Could you check a few things on this model? Use its own coordinates, in mm. A direction names the side the tool comes from. Round coordinates to 2 decimals unless told otherwise and drop trailing zeros. Loops run counter-clockwise (first coordinate to the right, second up) from the corner with the lowest first, then second, coordinate; pieces in that order, holes last.
from build123d import *

# Parameters (mm, degrees)
SKETCH_W        = 160
SKETCH_H        = 160
PAD_DEPTH       = 10
SKETCH001_R     = 80
SKETCH001_R_2   = 64
POCKET_DEPTH    = 5
SKETCH002_R     = 3.1
POCKET001_DEPTH = 10
SKETCH003_R     = 10
PAD001_DEPTH    = 10
SKETCH004_R     = 3.1
POCKET002_DEPTH = 14


with BuildPart() as part:
    # Sketch → Pad (new body)
    with BuildSketch(Plane.XY):
        with Locations((80, 80)):
            Rectangle(SKETCH_W, SKETCH_H)
    extrude(amount=PAD_DEPTH)

    # Sketch001 (on Face6 of Pad) → Pocket (cut)
    with BuildSketch(Plane.XY.offset(10)):
        with Locations((48, 48)):
            Circle(SKETCH001_R)
        with Locations((48, 48)):
            Circle(SKETCH001_R_2, mode=Mode.SUBTRACT)
    extrude(amount=-POCKET_DEPTH, mode=Mode.SUBTRACT)

    # Sketch002 (on Face5 of Pocket) → Pocket001 (cut)
    with BuildSketch(Plane.XY.offset(10)):
        with Locations((20, 140)):
            Circle(SKETCH002_R)
        with Locations((80, 140)):
            Circle(SKETCH002_R)
        with Locations((140, 140)):
            Circle(SKETCH002_R)
        with Locations((140, 80)):
            Circle(SKETCH002_R)
        with Locations((140, 20)):
            Circle(SKETCH002_R)
    extrude(amount=-POCKET001_DEPTH, mode=Mode.SUBTRACT)

    # Sketch003 (on Face9 of Pocket001) → Pad001 (join)
    with BuildSketch(Plane.XY.offset(10)):
        with Locations((48, 48)):
            Circle(SKETCH003_R)
    extrude(amount=PAD001_DEPTH)

    # Sketch004 (on Face21 of Pad001) → Pocket002 (cut)
    with BuildSketch(Plane.XY.offset(20)):
        with Locations((48, 48)):
            Circle(SKETCH004_R)
    extrude(amount=-POCKET002_DEPTH, mode=Mode.SUBTRACT)


solid = part.part
Item 1: We'd pull the mould along X, two halves only. Please class faces 1 (the cylindrical face through (142.957, 20.931, 5.07)), 2 (the flat face through (114, 117, 10)), 3 (the cylindrical face through (2.71, 2.78, 7.54)): released by +X, released by -X, zero draft, split by the parting line, or undercut.
Results list:
face 1: undercut
face 2: zero draft
face 3: released by -X
Item 2: Will these pins go through, and if not, where does the flat tip stop? pin 1 (7 mm diameter, centred on x = 49, y = 48, fed in from +Z); pin 2 (8 mm diameter, centred on x = 20, y = 140, fed in from +Z); pin 3 (1 mm diameter, centred on y = 56.5, z = 14.5, fed in from +X); pin 4 (5 mm diameter, centred on x = 140, y = 80, fed in from +Z).
Results list:
pin 1: stops at z = 20
pin 2: stops at z = 10
pin 3: stops at x = 54
pin 4: passes through
Item 3: If we section it at D-D, the plane x = 80: Please give me the cut outline in (y, z).
Results list:
outline: (0, 0) - (136.9, 0) - (136.9, 10) - (121.32, 10) - (121.32, 5) - (103.43, 5) - (103.43, 10) - (0, 10) - close; (143.1, 0) - (160, 0) - (160, 10) - (143.1, 10) - close
Item 4: If we section it at C-C, the plane y = 20: Please give me the cut outline in (x, z), then the cut area to 3 significant figures.
Results list:
outline: (0, 0) - (136.9, 0) - (136.9, 10) - (122.94, 10) - (122.94, 5) - (105.55, 5) - (105.55, 10) - (0, 10) - close; (143.1, 0) - (160, 0) - (160, 10) - (143.1, 10) - close
area: 1,450 mm2
Item 5: For faces 4 (the cylindrical face through (47.596, 51.074, 13.098)), 5 (the cylindrical face through (142.864, 78.813, 5.07)), which set-ups out of +Z, -Z, +X, -X, +Y, -Y let a thin tool reach every point of the face, with its end or its side?
Results list:
face 4: +Z
face 5: +Z, -Z
Item 6: If I drill on line 1 along Y through (x, z) = (139.5, 3.25); line 2 along X through (y, z) = (140, 2.25); line 3 along Y through (x, z) = (48, 14), over which ranges is the centre line in solid material (lowest first)?
Results list:
line 1: y = 0 to 16.94, 23.06 to 76.94, 83.06 to 136.94, 143.06 to 160
line 2: x = 0 to 16.9, 23.1 to 76.9, 83.1 to 136.9, 143.1 to 160
line 3: y = 38 to 44.9, 51.1 to 58
Item 7: If we section it at A-A, the plane y = 140: Please give me the cut outline in (x, z), then the cut area to 3 significant figures.
Results list:
outline: (0, 0) - (16.9, 0) - (16.9, 10) - (0, 10) - close; (23.1, 0) - (76.9, 0) - (76.9, 10) - (23.1, 10) - close; (83.1, 0) - (136.9, 0) - (136.9, 10) - (83.1, 10) - close; (143.1, 0) - (160, 0) - (160, 10) - (143.1, 10) - close
area: 1,410 mm2
